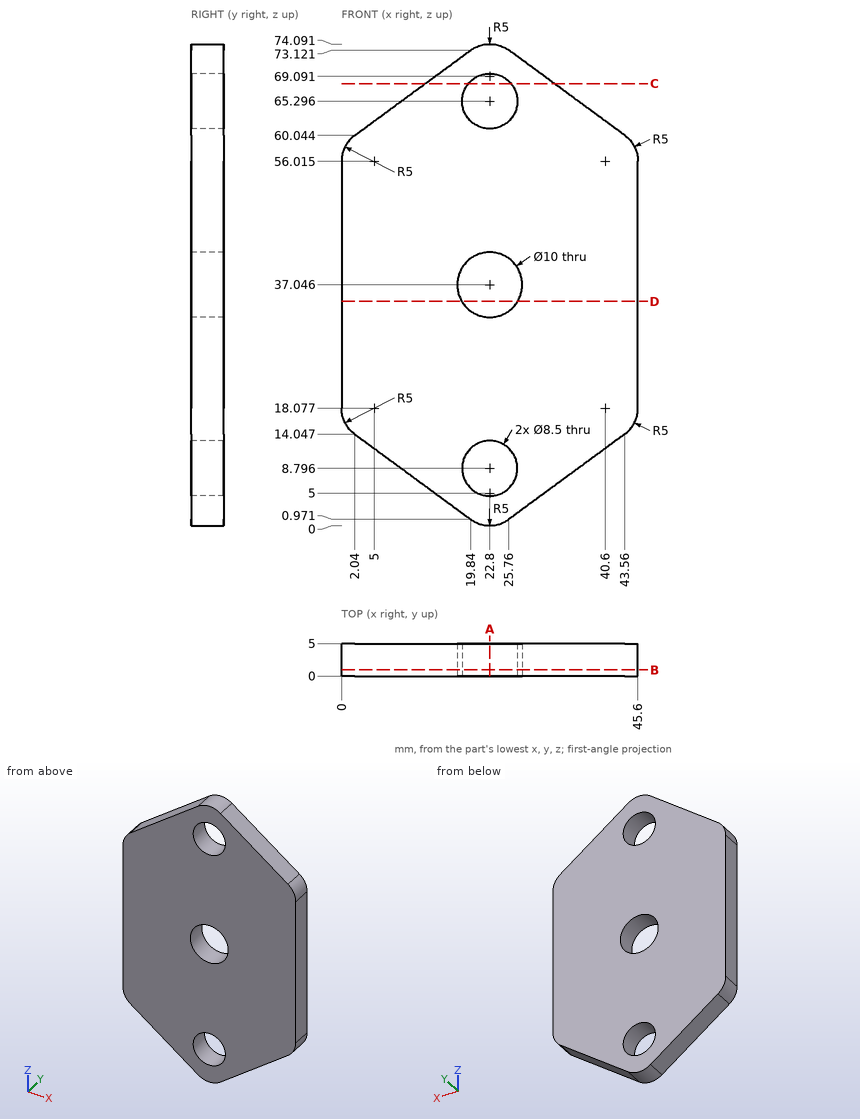
Design review of the part shown in the three views and the two pictorial views. Dimensions are in mm from the part's minimum x, y and z. Round coordinates to 2 decimals unless told otherwise and drop trailing zeros. Order: outer loops, then holes, each group sorted by start corner. A loop starts at its lowest first (then second) coordinate and runs counter-clockwise, first axis right, second up.
Item 1: Add section B-B, the plane y = 0.95. Count the separate pieces of the cut face and the enclosed holes in it, and give its area (3 significant figures).
Working result:
separate pieces: 1
enclosed holes: 3
area: 2,520 mm2
Item 2: For pin 1 (3 mm diameter, centred on x = 40, y = 0.5, fed in from -Z), flat-tipped, find the tip position at first contact; note if it passes through.
Working result:
pin 1: stops at z = 10.33
Item 3: Add section A-A, the plane x = 22.8. State the section outline as (y, z) points (1 decimal).
Working result:
outline: (0, 0) - (5, 0) - (5, 4.5) - (0, 4.5) - close; (0, 13) - (5, 13) - (5, 32) - (0, 32) - close; (0, 42) - (5, 42) - (5, 61) - (0, 61) - close; (0, 69.5) - (5, 69.5) - (5, 74.1) - (0, 74.1) - close
Item 4: Add section D-D, the plane z = 34.5. State the section outline as (x, y) points, and give its area (3 significant figures).
Working result:
outline: (0, 0) - (18.5, 0) - (18.5, 5) - (0, 5) - close; (27.1, 0) - (45.6, 0) - (45.6, 5) - (27.1, 5) - close
area: 185 mm2
Item 5: To check wall thickness, follow probe 1 along Z at (x, y) = (22.8, 3.5) (1 decimal); probe 2 along X at (y, z) = (4.1, 34) (1 decimal); probe 3 along X at (y, z) = (4.6, 10.5) (1 decimal). State the ranges of each line that lie inside material, in increasing order.
Working result:
probe 1: z = 0 to 4.5, 13 to 32, 42 to 61, 69.5 to 74.1
probe 2: x = 0 to 18.8, 26.8 to 45.6
probe 3: x = 6.9 to 18.9, 26.7 to 38.7
Item 6: Add section C-C, the plane z = 68. State the section outline as (x, y) points.
Working result:
outline: (12.87, 0) - (19.52, 0) - (19.52, 5) - (12.87, 5) - close; (26.08, 0) - (32.73, 0) - (32.73, 5) - (26.08, 5) - close
